Could you check a few things on this model? Use its own coordinates, in mm. Face numbers are marked on the shaded views. Give positions to 0.01 mm unless a question says otherwise; leave off trailing zeros. Loops run counter-clockwise (first coordinate to the right, second up) from the corner with the lowest first, then second, coordinate; pieces in that order, holes last. Notation, with made-up numbers: (-28, 60.5) - (27, 60.5) arc R21 cw to (27, 83.5) - close; hole circle Ø9 at (76.25, -23). An arc over 180 degrees is marked (long way). Write each question's results on one line, items separated by ' | '. Start each with the question number.
1) I want a section at A-A, the plane x = 0. Write out the boundary of the cut face in (y, z).
2) I'm going to push flat-ended pins straight in: pin 1 (2 mm diameter, centred on x = 10.5, z = 26, fed in from +Y); pin 2 (1.6 mm diameter, centred on x = 0, z = 60.5, fed in from +Y); pin 3 (1 mm diameter, centred on y = 18.5, z = 61.5, fed in from +X). Where does each tip first touch, or does it pass through?
3) I want a section at D-D, the plane z = 57. Write out the boundary of the cut face in (x, y).
4) If I drill on probe 1 along Y at (x, z) = (0, 38); probe 2 along X at (y, z) = (1.5, 9); probe 3 along Y at (x, z) = (-9.5, 45), over which ranges is the centre line in solid material (lowest first)? Write a range as [from, to].
5) I want a section at B-B, the plane y = 0. Write out the boundary of the cut face in (x, z).
6) I want a section at C-C, the plane z = 9. Write out the boundary of the cut face in (x, y).
7) If we mould it in two halves opening along Z, with no side actions, what happens to the marked faces 1, 2 and 3? For each: +Z half, -Z half, draft (parallel to the pull), parting line (faces both ways), or undercut.
from build123d import *

# Parameters (mm, degrees)
SKETCH2_R           = 22.5
SKETCH2_R_2         = 12.75
BOSS_EXTRUDE1_DEPTH = 60
SKETCH4_W           = 2.545484213
SKETCH4_H           = 3.916129558
BOSS_EXTRUDE2_DEPTH = 2


with BuildPart() as part:
    # Sketch2 → Boss-Extrude1 (new body)
    with BuildSketch(Plane.XY):
        Circle(SKETCH2_R)
        Circle(SKETCH2_R_2, mode=Mode.SUBTRACT)
    extrude(amount=BOSS_EXTRUDE1_DEPTH)

    # Sketch3 → Cut-Revolve1 (revolve, cut)
    with BuildSketch(Plane(origin=(0, 0, 0), x_dir=(1, 0, 0), z_dir=(0, 1, 0)), mode=Mode.PRIVATE) as cut_revolve1_sk:
        Polygon((22.5, -5), (22.5, -55), (15, -47.5), (15, -12.5), align=None)
    revolve(cut_revolve1_sk.sketch.rotate(Axis((0, 0, -10.796502134), (0, 0, 1)), 180), axis=Axis((0, 0, -10.796502134), (0, 0, 1)), mode=Mode.SUBTRACT)

    # Sketch4 → Boss-Extrude2 (add)
    with BuildSketch(Plane.XY.offset(60)):
        with Locations((-0.489516195, 17.557314188)):
            Rectangle(SKETCH4_W, SKETCH4_H)
    extrude(amount=BOSS_EXTRUDE2_DEPTH)


solid = part.part
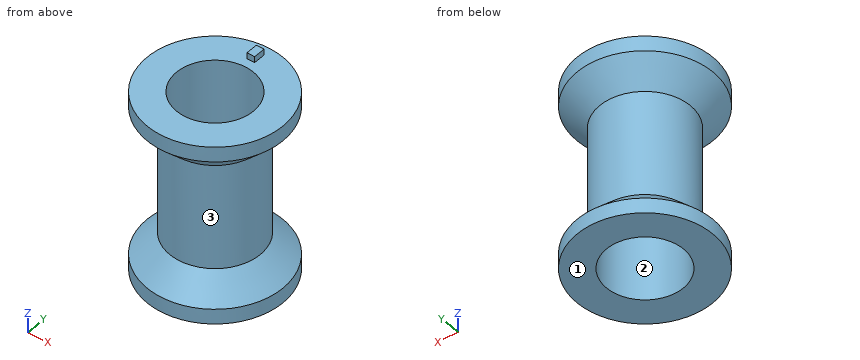
Answers:
1) outline: (-22.5, 0) - (-12.75, 0) - (-12.75, 60) - (-22.5, 60) - (-22.5, 55) - (-15, 47.5) - (-15, 12.5) - (-22.5, 5) - close; (12.75, 0) - (22.5, 0) - (22.5, 5) - (15, 12.5) - (15, 47.5) - (22.5, 55) - (22.5, 60) - (19.52, 60) - (19.52, 62) - (15.6, 62) - (15.6, 60) - (12.75, 60) - close
2) pin 1: stops at y = 11.61 | pin 2: stops at y = 22.5 | pin 3: stops at x = 0.78
3) outline: circle Ø45 at (0, 0); hole circle Ø25.5 at (0, 0)
4) probe 1: y = [-15, -12.75], [12.75, 15] | probe 2: x = [-18.44, -12.66], [12.66, 18.44] | probe 3: y = [-11.61, -8.5], [8.5, 11.61]
5) outline: (-22.5, 0) - (-12.75, 0) - (-12.75, 60) - (-22.5, 60) - (-22.5, 55) - (-15, 47.5) - (-15, 12.5) - (-22.5, 5) - close; (12.75, 0) - (22.5, 0) - (22.5, 5) - (15, 12.5) - (15, 47.5) - (22.5, 55) - (22.5, 60) - (12.75, 60) - close
6) outline: circle Ø37 at (0, 0); hole circle Ø25.5 at (0, 0)
7) face 1: -Z half | face 2: draft | face 3: undercut
